Geometry check sheet. Reference: drawing and pictorial views, mm from the part's lowest x, y, z. Round coordinates to 2 decimals unless told otherwise and drop trailing zeros. Write each loop counter-clockwise with the first axis right and the second up, starting at its lowest first coordinate (ties: lowest second). Pieces come first, ordered by that corner, then holes. Notation, with made-up numbers: M 64.5,18.5 L 114.5,18.5 A18 ccw 114.5,33.5 Z; hole C 88.5,36.25 d9. An arc over 180 degrees is marked long. Put each result on its own line as item: value. Start each with the question number.
(1) Material ranges on probe 1 along Y at (x, z) = (3, 2); probe 2 along X at (y, z) = (6, 2.05); probe 3 along X at (y, z) = (2.5, 3), recorded low to high.
(2) Section check C-C on z = 2.5. Record the cut outline in (x, y).
(3) Section check B-B on y = 24. Record the cut outline in (x, z), then the cut area to 3 significant figures.
(4) Section check D-D on x = 39. Record the cut outline in (y, z) (3 decimals), then the cut area to 3 significant figures.
(5) Section check A-A on x = 3. Record the cut outline in (y, z).
(6) Gauge pin test, flat end, axial feed: pin 1 (4 mm diameter, centred on x = 30.5, y = 6.5, fed in from -Z). Record the tip position at first contact, or that the pin passes through.
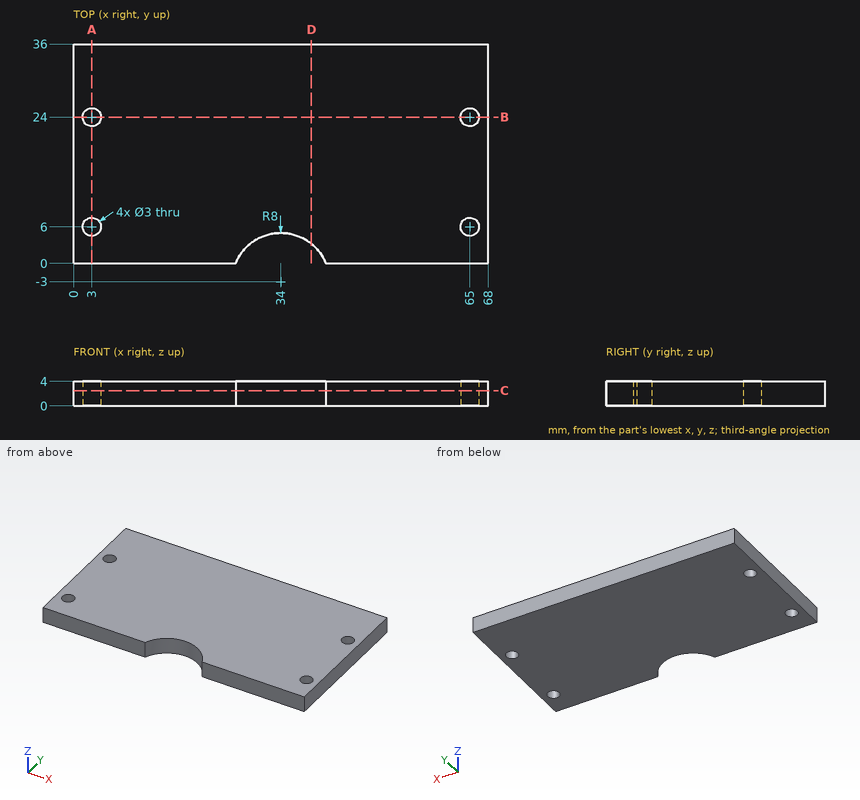
Answers follow:
1. probe 1: y = 0 to 4.5, 7.5 to 22.5, 25.5 to 36
1. probe 2: x = 0 to 1.5, 4.5 to 63.5, 66.5 to 68
1. probe 3: x = 0 to 28.19, 39.81 to 68
2. outline: M 0,0 L 26.58,0 A8 cw 41.42,0 L 68,0 L 68,36 L 0,36 Z; hole C 3,6 d3; hole C 3,24 d3; hole C 65,6 d3; hole C 65,24 d3
3. outline: M 0,0 L 1.5,0 L 1.5,4 L 0,4 Z; M 4.5,0 L 63.5,0 L 63.5,4 L 4.5,4 Z; M 66.5,0 L 68,0 L 68,4 L 66.5,4 Z
3. area: 248 mm^2
4. outline: M 3.245,0 L 36,0 L 36,4 L 3.245,4 Z
4. area: 131 mm^2
5. outline: M 0,0 L 4.5,0 L 4.5,4 L 0,4 Z; M 7.5,0 L 22.5,0 L 22.5,4 L 7.5,4 Z; M 25.5,0 L 36,0 L 36,4 L 25.5,4 Z
6. pin 1: stops at z = 0
